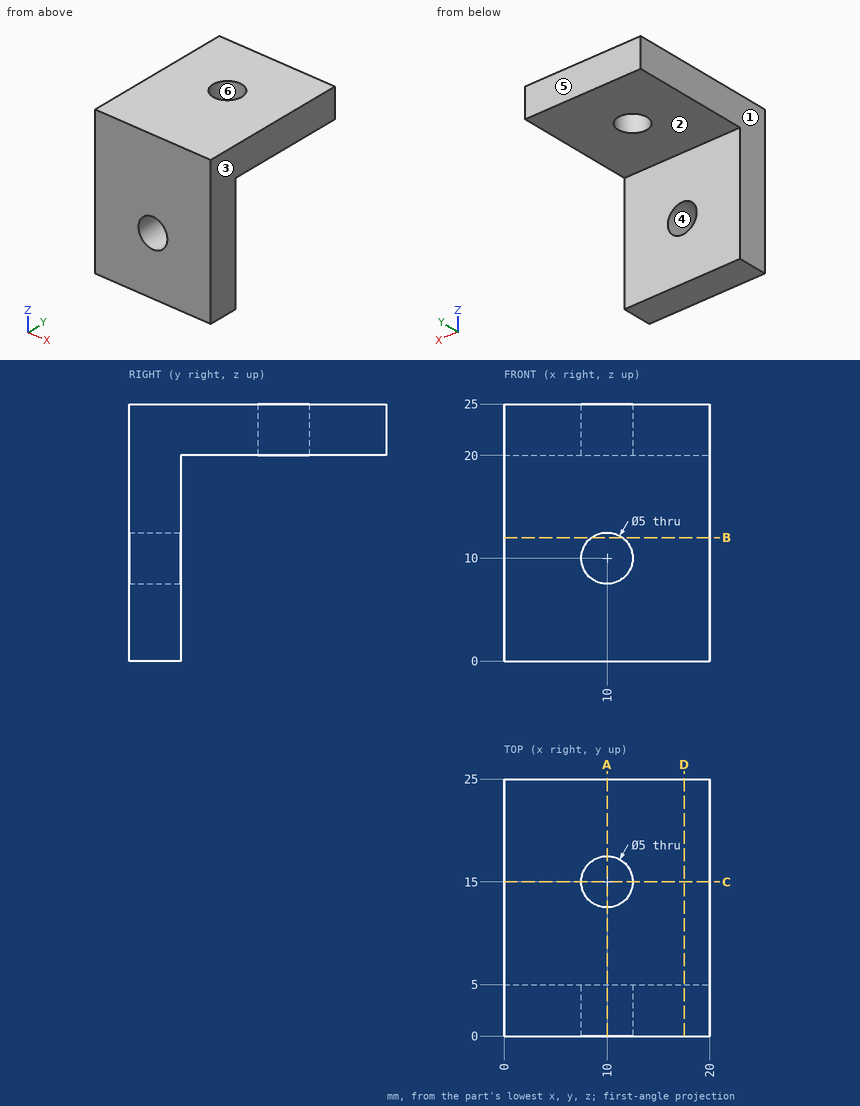
The figure shows three views and two pictorial views of one solid part (mm, origin at its lowest corner). Answer the questions. A direction names the side the tool comes from. Round coordinates to 2 decimals unless told otherwise and drop trailing zeros. Order: outer loops, then holes, each group sorted by start corner. A loop starts at its lowest first (then second) coordinate and runs counter-clockwise, first axis right, second up. Notation, with made-up numbers: (3.25, 54.5) -> (26.25, 54.5) arc R11 cw to (26.25, 68.5) -> close; hole circle Ø8 at (-32, -10.5). An arc over 180 degrees is marked (long way). One line per item, written item: value.
Item 1: Find section A-A, the plane x = 10. Give the vertices of the cut face in (y, z), then the cut area to 3 significant figures.
Taken from the geometry:
outline: (0, 0) -> (5, 0) -> (5, 7.5) -> (0, 7.5) -> close; (0, 12.5) -> (5, 12.5) -> (5, 20) -> (12.5, 20) -> (12.5, 25) -> (0, 25) -> close; (17.5, 20) -> (25, 20) -> (25, 25) -> (17.5, 25) -> close
area: 175 mm2
Item 2: Given P1, Ø10, axis at x = 6, z = 13, coming from the +Y side; P2, Ø8, axis at x = 11.5, y = 19, coming from the -Z side; P3, Ø3, axis at x = 10, z = 10, coming from the +Y side, each flat-ended and moving along its own axis, determine where each tip first touches the part or whether it passes through.
Taken from the geometry:
P1: stops at y = 5
P2: stops at z = 20
P3: passes through
Item 3: Find section D-D, the plane x = 17.5. Give the vertices of the cut face in (y, z), then the cut area to 3 significant figures.
Taken from the geometry:
outline: (0, 0) -> (5, 0) -> (5, 20) -> (25, 20) -> (25, 25) -> (0, 25) -> close
area: 225 mm2
Item 4: Straight lines are drawn through the part: L1, parallel to X at y = 1.45, z = 10; L2, parallel to Z at x = 10, y = 3.6; L3, parallel to Z at x = 11, y = 7.5. For each, find the intervals that lie inside material, in ascending order.
Taken from the geometry:
L1: x = 0 to 7.5, 12.5 to 20
L2: z = 0 to 7.5, 12.5 to 25
L3: z = 20 to 25
Item 5: For the marked faces 1 and 2, determine the directions among +Z, -Z, +X, -X, +Y, -Y from which every point of the face is accessible in a straight line to the end or side of a thin tool.
Taken from the geometry:
face 1: +Z, -Z, -X, +Y, -Y
face 2: -Z, +X, -X, +Y
Item 6: For a pull along X with two mould halves and no side action, classify the marked faces 3, 4, 5 and 6 as released by +X, released by -X, zero draft, split by the parting line, or undercut.
Taken from the geometry:
face 3: released by +X
face 4: undercut
face 5: zero draft
face 6: undercut
Item 7: Find section C-C, the plane y = 15. Give the vertices of the cut face in (x, z), then the cut area to 3 significant figures.
Taken from the geometry:
outline: (0, 20) -> (7.5, 20) -> (7.5, 25) -> (0, 25) -> close; (12.5, 20) -> (20, 20) -> (20, 25) -> (12.5, 25) -> close
area: 75.0 mm2
Item 8: Find section B-B, the plane z = 12. Give the vertices of the cut face in (x, y).
Taken from the geometry:
outline: (0, 0) -> (8.5, 0) -> (8.5, 5) -> (0, 5) -> close; (11.5, 0) -> (20, 0) -> (20, 5) -> (11.5, 5) -> close
